```python
from build123d import *

# Parameters (mm, degrees)
RESSALTO_EXTRUS_O1_DEPTH      = 3
ESBO_O1_3_W                   = 16.6
ESBO_O1_3_H                   = 23
ESBO_O1_3_R                   = 2
ESBO_O1_3_R_2                 = 0.5
RESSALTO_EXTRUS_O2_DEPTH      = 6
CORTE_EXTRUS_O1_DEPTH         = 3
CORTE_EXTRUS_O2_DEPTH         = 29.522973197
CHANFRO1_SIZE                 = 6
FURO_ROSCADO_DE_M3X0_51_D     = 2.5
FURO_ROSCADO_DE_M3X0_51_DEPTH = 8.5
FURO_ROSCADO_DE_M3X0_51_TIP   = 0.751075774
FURO_ROSCADO_DE_M3X0_52_D     = 2.5
FURO_ROSCADO_DE_M3X0_53_D     = 2.5
FURO_ROSCADO_DE_M3X0_53_DEPTH = 3
FURO_ROSCADO_DE_M3X0_53_TIP   = 0.751075774
ESBO_O18_R                    = 2.45
RESSALTO_EXTRUS_O3_DEPTH      = 3.5
CHANFRO2_SIZE                 = 0.5
FURO_ROSCADO_DE_M5X0_81_D     = 4.2
FURO_ROSCADO_DE_M5X0_81_DEPTH = 14
FURO_ROSCADO_DE_M5X0_81_TIP   = 1.2618073


with BuildPart() as part:
    # Esboço1 → Ressalto-extrusão1 (new body)
    with BuildSketch(Plane.XY):
        with BuildLine():
            Line((0, -2), (0, 0))
            Line((0, 0), (0, 16))
            ThreePointArc((0, 16), (-1.757359313, 11.757359313), (-6, 10))
            ThreePointArc((-6, 10), (-12, 4), (-6, -2))
            Line((-6, -2), (0, -2))
        make_face()
    extrude(amount=RESSALTO_EXTRUS_O1_DEPTH)

    # Esboço1<3> → Ressalto-extrusão2 (add)
    with BuildSketch(Plane.XY):
        with Locations((8.3, 11.5)):
            Rectangle(ESBO_O1_3_W, ESBO_O1_3_H)
        with Locations((11.6, 17.6)):
            Circle(ESBO_O1_3_R, mode=Mode.SUBTRACT)
        with Locations((4.68, 17.61)):
            Circle(ESBO_O1_3_R_2, mode=Mode.SUBTRACT)
    extrude(amount=RESSALTO_EXTRUS_O2_DEPTH)

    # Esboço2 → Corte-extrusão1 (cut)
    with BuildSketch(Plane.XY.offset(6)):
        Polygon((0, 3.633024279), (2.37796561, 23), (0, 23), align=None)
    extrude(amount=-CORTE_EXTRUS_O1_DEPTH, mode=Mode.SUBTRACT)

    # Esboço3 → Corte-extrusão2 (cut, through all)
    with BuildSketch(Plane.XY.offset(3)):
        with BuildLine():
            ThreePointArc((-6, 10), (-5.633708763, 9.988808791), (-5.26878394, 9.95527691))
            Line((-5.26878394, 9.95527691), (0.68649297, 9.224060849))
            Line((0.68649297, 9.224060849), (2.37796561, 23))
            Line((2.37796561, 23), (0, 23))
            Line((0, 23), (0, 16))
            ThreePointArc((0, 16), (-1.757359313, 11.757359313), (-6, 10))
        make_face()
    extrude(amount=-CORTE_EXTRUS_O2_DEPTH, mode=Mode.SUBTRACT)

    # Chanfro1
    # the kernel refuses this chamfer: 6 mm, written as the material it adds along each edge
    with BuildSketch(Plane(origin=(0.68649297, 9.224060849, 3), x_dir=(-0.9955217911555101, 0.09453234015153283, 0), z_dir=(0, 0, -1))) as chanfro1_piece_1:
        Polygon((CHANFRO1_SIZE * 0.999621916911, CHANFRO1_SIZE * 0.0274958766106), (-CHANFRO1_SIZE * 0.0274958766106, CHANFRO1_SIZE * 0.999621916911), (0, 0), align=None)
    extrude(amount=3)

    # Furo roscado de M3x0.51
    with Locations(Plane.XZ):
        with Locations((4, 3), (12.6, 3)):
            Hole(FURO_ROSCADO_DE_M3X0_51_D / 2, depth=FURO_ROSCADO_DE_M3X0_51_DEPTH)
            with Locations((0, 0, -(FURO_ROSCADO_DE_M3X0_51_DEPTH + FURO_ROSCADO_DE_M3X0_51_TIP / 2))):  # 118° drill point
                Cone(0, FURO_ROSCADO_DE_M3X0_51_D / 2, FURO_ROSCADO_DE_M3X0_51_TIP, mode=Mode.SUBTRACT)

    # Furo roscado de M3x0.52 (through all)
    with Locations(Plane.XY.offset(6)):
        with Locations((4.68, 17.61)):
            Hole(FURO_ROSCADO_DE_M3X0_52_D / 2)

    # Furo roscado de M3x0.53
    with Locations(Plane(origin=(0, 23, 0), x_dir=(1, 0, 0), z_dir=(0, 1, 0))):
        with Locations((8.1, -3)):
            Hole(FURO_ROSCADO_DE_M3X0_53_D / 2, depth=FURO_ROSCADO_DE_M3X0_53_DEPTH)
            with Locations((0, 0, -(FURO_ROSCADO_DE_M3X0_53_DEPTH + FURO_ROSCADO_DE_M3X0_53_TIP / 2))):  # 118° drill point
                Cone(0, FURO_ROSCADO_DE_M3X0_53_D / 2, FURO_ROSCADO_DE_M3X0_53_TIP, mode=Mode.SUBTRACT)

    # Esboço18 → Ressalto-extrusão3 (add)
    with BuildSketch(Plane.XY.offset(3)):
        with Locations((-6, 4)):
            Circle(ESBO_O18_R)
    extrude(amount=RESSALTO_EXTRUS_O3_DEPTH)

    # Chanfro2
    chanfro2_edges = [part.edges().sort_by_distance(p)[0] for p in [
        (-8.45, 4, 6.5),
    ]]
    chamfer(chanfro2_edges, length=CHANFRO2_SIZE)

    # Furo roscado de M5x0.81
    with Locations(Plane.XY.offset(6)):
        with Locations((11.6, 17.6)):
            Hole(FURO_ROSCADO_DE_M5X0_81_D / 2, depth=FURO_ROSCADO_DE_M5X0_81_DEPTH)
            with Locations((0, 0, -(FURO_ROSCADO_DE_M5X0_81_DEPTH + FURO_ROSCADO_DE_M5X0_81_TIP / 2))):  # 118° drill point
                Cone(0, FURO_ROSCADO_DE_M5X0_81_D / 2, FURO_ROSCADO_DE_M5X0_81_TIP, mode=Mode.SUBTRACT)


solid = part.part
```
Source: CAD feature listing. Evaluate the final solid. Frame: model axes, mm. A direction names the side the tool comes from. Coordinates: 2 decimals unless noted, no trailing zeros. Write each loop counter-clockwise with the first axis right and the second up, starting at its lowest first coordinate (ties: lowest second). Pieces come first, ordered by that corner, then holes. Notation, with made-up numbers: (89, -27) - (146, -27) arc R3 cw to (146, -23) - close; hole circle Ø5 at (27, 24). An arc over 180 degrees is marked (long way). Answer as a JSON object with one key per item and string values.
Q1. First-contact query: pin 1 Ø0.9 at (y, z) = (2, 5) entering from -X; pin 2 Ø1.6 at (y, z) = (-1, 1.5) entering from +X; pin 3 Ø1.5 at (x, y) = (2, 6) entering from +Z. Flat tips, straight axial feed; report the tip coordinate or a pass-through.
Ans:
{"pin 1": "stops at x = -7.9", "pin 2": "stops at x = 0", "pin 3": "stops at z = 6"}
Q2. Material intervals for line 1 (Z direction, x = 8.1, y = 21.6); line 2 (Y direction, x = 4.68, z = 4.75); line 3 (Z direction, x = -2.25, y = 9.75), sorted ascending. Write a range as [from, to].
Ans:
{"line 1": "z = [0, 1.75], [4.25, 6]", "line 2": "y = [0, 16.36], [18.86, 23]", "line 3": "z = [0, 3]"}
Q3. Section query C-C, the plane x = -9.25. Output: boundary loops of the cut face in (y, z), plus the area to 3 significant figures.
Ans:
{"outline": "(-1.04, 0) - (9.04, 0) - (9.04, 3) - (-1.04, 3) - close", "area": "30.3 mm2"}
Q4. Section query A-A, the plane y = 4. Output: boundary loops of the cut face in (x, z), plus the area to 3 significant figures.
Ans:
{"outline": "(-12, 0) - (16.6, 0) - (16.6, 6) - (0.05, 6) - (0.05, 3) - (-3.55, 3) - (-3.55, 6) - (-4.05, 6.5) - (-7.95, 6.5) - (-8.45, 6) - (-8.45, 3) - (-12, 3) - close; hole circle Ø2.5 at (4, 3); hole circle Ø2.5 at (12.6, 3)", "area": "143 mm2"}
Q5. Set-up query: faces 4 (the flat face through (-3, 5, 3)), 5 (the flat face through (8, 0, 3)), 6 (the cylindrical face through (4.921, 4.31, 3.845)), 7 (the cylindrical face through (9.021, 21.479, 2.155)), 8 (the flat face through (0, 2, 4)). Return all of +Z, -Z, +X, -X, +Y, -Y with unobstructed straight access to the full face (end or side cutting, diameter ignored); none if empty.
Ans:
{"face 4": "+Z", "face 5": "+Z, -Z, +X, -Y", "face 6": "-Y", "face 7": "+Y", "face 8": "+Z, +Y, -Y"}
Q6. Section query B-B, the plane y = 14.25. Output: boundary loops of the cut face in (x, z).
Ans:
{"outline": "(0.23, 0) - (16.6, 0) - (16.6, 6) - (1.3, 6) - (1.3, 3) - (0.23, 3) - close"}
Q7. Draft query along X for faces 1 (the conical face through (12.44, 9.12, 3.15)), 2 (the flat face through (8, 12, 6)), 3 (the flat face through (0, -1, 1)). Return one class per face: released by +X, released by -X, zero draft, split by the parting line, or undercut.
Ans:
{"face 1": "undercut", "face 2": "zero draft", "face 3": "released by +X"}
